Build history of the part. All positions in model axes, mm. A direction names the side the tool comes from. Round coordinates to 2 decimals unless told otherwise and drop trailing zeros. Order: outer loops, then holes, each group sorted by start corner. A loop starts at its lowest first (then second) coordinate and runs counter-clockwise, first axis right, second up. Notation, with made-up numbers: (35, -38.5) -> (67, -38.5) arc R23 cw to (67, -23.5) -> close; hole circle Ø8 at (68, -40). An arc over 180 degrees is marked (long way). Use a Markdown table: item, result. Add a question column.
Item 1: Slice it at B-B, the plane y = 18.5. Give the cut face in (x, z).
Item 2: Slice it at D-D, the plane z = 44.5. Give the cut face in (x, y), plus the area to 3 significant figures.
Item 3: Slice it at A-A, the plane y = 3. Give the cut face in (x, z), plus the area to 3 significant figures.
Item 4: 3-axis set-ups, long thin cutter, end or side, ignore diameter. For faces 4 (the face through (-37, 13, 52.589)), 5 (the face through (-11, 13, 17)), 6 (the face through (-69.738, 2.465, 65.537)): which of +Z, -Z, +X, -X, +Y, -Y reach the whole face in a straight line?
Item 5: Two-plate mould, pull along Z, no slides. Class faces 1 (the face through (-38, 20, 6)), 2 (the face through (-38, 10, -8.411)), 3 (the face through (-71.893, 2, 21)): released by +Z, released by -Z, zero draft, split by the parting line, or undercut.
Item 6: Pin check, flat tips, straight feed: pin 1 (11.5 mm diameter, centred on x = -7.64, z = 21.34, fed in from +Y); pin 2 (3.5 mm diameter, centred on x = -7.64, z = 21.34, fed in from +Y); pin 3 (4.5 mm diameter, centred on x = -8, z = 61, fed in from -Y). Stop position of each tip, or through.
Item 7: Probe L1, parallel to X at y = 2.75, z = 64; L2, parallel to Z at x = -71, y = 2.5; L3, parallel to X at y = 16, z = 11.5. List the from-to ranges inside material, lowest first.
Item 8: Slice it at C-C, the plane x = -46. Give the cut face in (y, z), plus the area to 3 significant figures.
from build123d import *

# Parameters (mm, degrees)
SKETCH2_W           = 100
SKETCH2_H           = 100
BOSS_EXTRUDE1_DEPTH = 20
SKETCH3_W           = 100
SKETCH3_H           = 20
CUT_EXTRUDE1_DEPTH  = 12
SKETCH5_R           = 13
CUT_EXTRUDE2_DEPTH  = 7
SKETCH6_R           = 13
CUT_EXTRUDE3_DEPTH  = 7
SKETCH8_R           = 13
CUT_EXTRUDE5_DEPTH  = 7
SKETCH7_R           = 13
CUT_EXTRUDE10_DEPTH = 7
SKETCH13_R          = 2.75
CUT_EXTRUDE11_DEPTH = 128.4313455
SKETCH14_R          = 2.75
CUT_EXTRUDE12_DEPTH = 128.4313455
SKETCH15_R          = 2.75
CUT_EXTRUDE13_DEPTH = 128.4313455
SKETCH16_R          = 2.75
CUT_EXTRUDE14_DEPTH = 128.4313455
CUT_EXTRUDE15_DEPTH = 5
CUT_EXTRUDE16_DEPTH = 5
CUT_EXTRUDE17_DEPTH = 5
CUT_EXTRUDE18_DEPTH = 5
SKETCH22_W          = 100
SKETCH22_H          = 12
CUT_EXTRUDE19_DEPTH = 1
SKETCH23_W          = 100
SKETCH23_H          = 12
CUT_EXTRUDE20_DEPTH = 1
SKETCH24_R          = 5
CUT_EXTRUDE21_DEPTH = 5
SKETCH25_R          = 5
CUT_EXTRUDE22_DEPTH = 5
SKETCH26_R          = 5
CUT_EXTRUDE23_DEPTH = 5
SKETCH27_R          = 5
CUT_EXTRUDE24_DEPTH = 5


with BuildPart() as part:
    # Sketch2 → Boss-Extrude1 (new body)
    with BuildSketch(Plane(origin=(0, 0, 0), x_dir=(1, 0, 0), z_dir=(0, 1, 0))):
        with Locations((-37.64268429, -41.588796838)):
            Rectangle(SKETCH2_W, SKETCH2_H)
    extrude(amount=BOSS_EXTRUDE1_DEPTH)

    # Sketch3 → Cut-Extrude1 (cut)
    with BuildSketch(Plane(origin=(0, 20, 0), x_dir=(1, 0, 0), z_dir=(0, 1, 0))):
        with Locations((-37.64268429, -41.588796838)):
            Rectangle(SKETCH3_W, SKETCH3_H)
    extrude(amount=-CUT_EXTRUDE1_DEPTH, mode=Mode.SUBTRACT)

    # Sketch5 → Cut-Extrude2 (cut)
    with BuildSketch(Plane(origin=(0, 20, 0), x_dir=(1, 0, 0), z_dir=(0, 1, 0))):
        with Locations((-7.64268429, -61.838796838)):
            Circle(SKETCH5_R)
    extrude(amount=-CUT_EXTRUDE2_DEPTH, mode=Mode.SUBTRACT)

    # Sketch6 → Cut-Extrude3 (cut)
    with BuildSketch(Plane(origin=(0, 20, 0), x_dir=(1, 0, 0), z_dir=(0, 1, 0))):
        with Locations((-67.64268429, -61.838796838)):
            Circle(SKETCH6_R)
    extrude(amount=-CUT_EXTRUDE3_DEPTH, mode=Mode.SUBTRACT)

    # Sketch8 → Cut-Extrude5 (cut)
    with BuildSketch(Plane(origin=(0, 20, 0), x_dir=(1, 0, 0), z_dir=(0, 1, 0))):
        with Locations((-7.64268429, -21.338796838)):
            Circle(SKETCH8_R)
    extrude(amount=-CUT_EXTRUDE5_DEPTH, mode=Mode.SUBTRACT)

    # Sketch7 → Cut-Extrude10 (cut)
    with BuildSketch(Plane(origin=(0, 20, 0), x_dir=(1, 0, 0), z_dir=(0, 1, 0))):
        with Locations((-67.64268429, -21.338796838)):
            Circle(SKETCH7_R)
    extrude(amount=-CUT_EXTRUDE10_DEPTH, mode=Mode.SUBTRACT)

    # Sketch13 → Cut-Extrude11 (cut, through all)
    with BuildSketch(Plane(origin=(0, 13, 0), x_dir=(1, 0, 0), z_dir=(0, 1, 0))):
        with Locations(Location((-67.64268429, -21.338796838, 0), (0, 0, 270))):
            Circle(SKETCH13_R)
    extrude(amount=-CUT_EXTRUDE11_DEPTH, mode=Mode.SUBTRACT)

    # Sketch14 → Cut-Extrude12 (cut, through all)
    with BuildSketch(Plane(origin=(0, 13, 0), x_dir=(1, 0, 0), z_dir=(0, 1, 0))):
        with Locations(Location((-7.64268429, -21.338796838, 0), (0, 0, 270))):
            Circle(SKETCH14_R)
    extrude(amount=-CUT_EXTRUDE12_DEPTH, mode=Mode.SUBTRACT)

    # Sketch15 → Cut-Extrude13 (cut, through all)
    with BuildSketch(Plane(origin=(0, 13, 0), x_dir=(1, 0, 0), z_dir=(0, 1, 0))):
        with Locations(Location((-7.64268429, -61.838796838, 0), (0, 0, 270))):
            Circle(SKETCH15_R)
    extrude(amount=-CUT_EXTRUDE13_DEPTH, mode=Mode.SUBTRACT)

    # Sketch16 → Cut-Extrude14 (cut, through all)
    with BuildSketch(Plane(origin=(0, 13, 0), x_dir=(1, 0, 0), z_dir=(0, 1, 0))):
        with Locations(Location((-67.64268429, -61.838796838, 0), (0, 0, 270))):
            Circle(SKETCH16_R)
    extrude(amount=-CUT_EXTRUDE14_DEPTH, mode=Mode.SUBTRACT)

    # Sketch17 → Cut-Extrude15 (cut)
    with BuildSketch(Plane(origin=(0, 0, 0), x_dir=(-1, 0, 0), z_dir=(0, -1, 0))):
        Polygon((7.64268429, -26.246274126), (11.89268429, -23.792535482), (11.89268429, -18.885058194), (7.64268429, -16.43131955), (3.39268429, -18.885058194), (3.39268429, -23.792535482), align=None)
    extrude(amount=-CUT_EXTRUDE15_DEPTH, mode=Mode.SUBTRACT)

    # Sketch19 → Cut-Extrude16 (cut)
    with BuildSketch(Plane.XZ):
        Polygon((-67.64268429, 26.246274126), (-71.89268429, 23.792535482), (-71.89268429, 18.885058194), (-67.64268429, 16.43131955), (-63.39268429, 18.885058194), (-63.39268429, 23.792535482), align=None)
    extrude(amount=-CUT_EXTRUDE16_DEPTH, mode=Mode.SUBTRACT)

    # Sketch20 → Cut-Extrude17 (cut)
    with BuildSketch(Plane.XZ):
        Polygon((-67.64268429, 66.746274126), (-71.89268429, 64.292535482), (-71.89268429, 59.385058194), (-67.64268429, 56.93131955), (-63.39268429, 59.385058194), (-63.39268429, 64.292535482), align=None)
    extrude(amount=-CUT_EXTRUDE17_DEPTH, mode=Mode.SUBTRACT)

    # Sketch21 → Cut-Extrude18 (cut)
    with BuildSketch(Plane.XZ):
        Polygon((-7.64268429, 66.746274126), (-11.89268429, 64.292535482), (-11.89268429, 59.385058194), (-7.64268429, 56.93131955), (-3.39268429, 59.385058194), (-3.39268429, 64.292535482), align=None)
    extrude(amount=-CUT_EXTRUDE18_DEPTH, mode=Mode.SUBTRACT)

    # Sketch22 → Cut-Extrude19 (cut)
    with BuildSketch(Plane.XY.offset(31.588796838)):
        with Locations((-37.64268429, 14)):
            Rectangle(SKETCH22_W, SKETCH22_H)
    extrude(amount=-CUT_EXTRUDE19_DEPTH, mode=Mode.SUBTRACT)

    # Sketch23 → Cut-Extrude20 (cut)
    with BuildSketch(Plane(origin=(0, 0, 51.588796838), x_dir=(-1, 0, 0), z_dir=(0, 0, -1))):
        with Locations((37.64268429, 14)):
            Rectangle(SKETCH23_W, SKETCH23_H)
    extrude(amount=-CUT_EXTRUDE20_DEPTH, mode=Mode.SUBTRACT)

    # Sketch24 → Cut-Extrude21 (cut)
    with BuildSketch(Plane(origin=(0, 13, 0), x_dir=(1, 0, 0), z_dir=(0, 1, 0))):
        with Locations(Location((-67.64268429, -61.838796838, 0), (0, 0, 270))):
            Circle(SKETCH24_R)
    extrude(amount=-CUT_EXTRUDE21_DEPTH, mode=Mode.SUBTRACT)

    # Sketch25 → Cut-Extrude22 (cut)
    with BuildSketch(Plane(origin=(0, 13, 0), x_dir=(1, 0, 0), z_dir=(0, 1, 0))):
        with Locations(Location((-7.64268429, -61.838796838, 0), (0, 0, 270))):
            Circle(SKETCH25_R)
    extrude(amount=-CUT_EXTRUDE22_DEPTH, mode=Mode.SUBTRACT)

    # Sketch26 → Cut-Extrude23 (cut)
    with BuildSketch(Plane(origin=(0, 13, 0), x_dir=(1, 0, 0), z_dir=(0, 1, 0))):
        with Locations(Location((-7.64268429, -21.338796838, 0), (0, 0, 270))):
            Circle(SKETCH26_R)
    extrude(amount=-CUT_EXTRUDE23_DEPTH, mode=Mode.SUBTRACT)

    # Sketch27 → Cut-Extrude24 (cut)
    with BuildSketch(Plane(origin=(0, 13, 0), x_dir=(1, 0, 0), z_dir=(0, 1, 0))):
        with Locations(Location((-67.64268429, -21.338796838, 0), (0, 0, 270))):
            Circle(SKETCH27_R)
    extrude(amount=-CUT_EXTRUDE24_DEPTH, mode=Mode.SUBTRACT)


solid = part.part
Check sheet entries:
| question | item | result |
|---|---|---|
| 1 | outline | (-87.64, -8.41) -> (12.36, -8.41) -> (12.36, 30.59) -> (1.49, 30.59) arc R13 cw (long way) to (-16.78, 30.59) -> (-58.51, 30.59) arc R13 cw (long way) to (-76.78, 30.59) -> (-87.64, 30.59) -> close; (-87.64, 52.59) -> (-76.78, 52.59) arc R13 cw (long way) to (-58.51, 52.59) -> (-16.78, 52.59) arc R13 cw (long way) to (1.49, 52.59) -> (12.36, 52.59) -> (12.36, 91.59) -> (-87.64, 91.59) -> close |
| 2 | outline | (-87.64, 0) -> (12.36, 0) -> (12.36, 8) -> (-87.64, 8) -> close |
| 2 | area | 800 mm2 |
| 3 | outline | (-87.64, -8.41) -> (12.36, -8.41) -> (12.36, 91.59) -> (-87.64, 91.59) -> close; hole (-71.89, 18.89) -> (-67.64, 16.43) -> (-63.39, 18.89) -> (-63.39, 23.79) -> (-67.64, 26.25) -> (-71.89, 23.79) -> close; hole (-71.89, 59.39) -> (-67.64, 56.93) -> (-63.39, 59.39) -> (-63.39, 64.29) -> (-67.64, 66.75) -> (-71.89, 64.29) -> close; hole (-11.89, 18.89) -> (-7.64, 16.43) -> (-3.39, 18.89) -> (-3.39, 23.79) -> (-7.64, 26.25) -> (-11.89, 23.79) -> close; hole (-11.89, 59.39) -> (-7.64, 56.93) -> (-3.39, 59.39) -> (-3.39, 64.29) -> (-7.64, 66.75) -> (-11.89, 64.29) -> close |
| 3 | area | 9,750 mm2 |
| 4 | face 4 | +X, -X, +Y |
| 4 | face 5 | +Y |
| 4 | face 6 | -Y |
| 5 | face 1 | zero draft |
| 5 | face 2 | released by -Z |
| 5 | face 3 | undercut |
| 6 | pin 1 | y = 13 |
| 6 | pin 2 | through |
| 6 | pin 3 | y = 5 |
| 7 | L1 | -87.64 to -71.89, -63.39 to -11.89, -3.39 to 12.36 |
| 7 | L2 | -8.41 to 18.37, 24.31 to 58.87, 64.81 to 91.59 |
| 7 | L3 | -87.64 to -76.14, -59.15 to -16.14, 0.85 to 12.36 |
| 8 | outline | (0, -8.41) -> (20, -8.41) -> (20, 30.59) -> (8, 30.59) -> (8, 52.59) -> (20, 52.59) -> (20, 91.59) -> (0, 91.59) -> close |
| 8 | area | 1,740 mm2 |
